Check sheet for the modelled part. Datum: model origin and axes. Units: mm. A direction names the side the tool comes from. Give positions to 0.01 mm unless a question says otherwise; leave off trailing zeros. Write each loop counter-clockwise with the first axis right and the second up, starting at its lowest first coordinate (ties: lowest second). Pieces come first, ordered by that corner, then holes. Notation, with made-up numbers: (53.5, 31) -> (74.5, 31) arc R17 ccw to (74.5, 35) -> close; hole circle Ø11 at (-9, -35). An arc over 180 degrees is marked (long way). Return JSON: item names as keys, results as strings.
from build123d import *

# Parameters (mm, degrees)
F1_DEPTH  = 26
F3_DEPTH  = 23
F4_W      = 86
F4_H      = 66
F5_DEPTH  = 5
F6_R      = 3
F7_R      = 3
F9_R      = 0.95
F10_DEPTH = 6


with BuildPart() as f1:
    # F0 (on Top) → F1 (new body)
    with BuildSketch(Plane.XY):
        with BuildLine():
            Line((76, 0), (10, 0))
            ThreePointArc((10, 0), (2.928932, -2.928932), (0, -10))
            Line((0, -10), (0, -56))
            ThreePointArc((0, -56), (2.928932, -63.071068), (10, -66))
            Line((10, -66), (76, -66))
            ThreePointArc((76, -66), (83.071068, -63.071068), (86, -56))
            Line((86, -56), (86, -10))
            ThreePointArc((86, -10), (83.071068, -2.928932), (76, 0))
        make_face()
    extrude(amount=F1_DEPTH)

    # F2 (on face) → F3 (cut)
    with BuildSketch(Plane.XY.offset(26)):
        with BuildLine():
            Line((73, -3), (13, -3))
            ThreePointArc((13, -3), (5.928932, -5.928932), (3, -13))
            Line((3, -13), (3, -53))
            ThreePointArc((3, -53), (5.928932, -60.071068), (13, -63))
            Line((13, -63), (73, -63))
            ThreePointArc((73, -63), (80.071068, -60.071068), (83, -53))
            Line((83, -53), (83, -13))
            ThreePointArc((83, -13), (80.071068, -5.928932), (73, -3))
        make_face()
    extrude(amount=-F3_DEPTH, mode=Mode.SUBTRACT)

    # F4 (on face) → F5 (cut)
    with BuildSketch(Plane.XY.offset(26)):
        with Locations((43, -33)):
            Rectangle(F4_W, F4_H)
        with BuildLine():
            ThreePointArc((1.5, -11.5), (4.428932, -4.428932), (11.5, -1.5))
            Line((11.5, -1.5), (74.5, -1.5))
            ThreePointArc((74.5, -1.5), (81.571068, -4.428932), (84.5, -11.5))
            Line((84.5, -11.5), (84.5, -54.5))
            ThreePointArc((84.5, -54.5), (81.571068, -61.571068), (74.5, -64.5))
            Line((74.5, -64.5), (11.5, -64.5))
            ThreePointArc((11.5, -64.5), (4.428932, -61.571068), (1.5, -54.5))
            Line((1.5, -54.5), (1.5, -11.5))
        make_face(mode=Mode.SUBTRACT)
    extrude(amount=-F5_DEPTH, mode=Mode.SUBTRACT)

    # F6
    f6_edges = [f1.edges().sort_by_distance(p)[0] for p in [
        (83.071068, -2.928932, 0),
        (43, 0, 0),
        (2.928932, -2.928932, 0),
        (0, -33, 0),
        (2.928932, -63.071068, 0),
        (43, -66, 0),
        (83.071068, -63.071068, 0),
        (86, -33, 0),
    ]]
    fillet(f6_edges, radius=F6_R)

    # F7
    f7_edges = [f1.edges().sort_by_distance(p)[0] for p in [
        (43, -3, 3),
        (5.928932, -5.928932, 3),
        (3, -33, 3),
        (5.928932, -60.071068, 3),
        (43, -63, 3),
        (80.071068, -60.071068, 3),
        (83, -33, 3),
        (80.071068, -5.928932, 3),
    ]]
    fillet(f7_edges, radius=F7_R)

    # F9 (on offset) → F10 (cut, symmetric)
    with BuildSketch(Plane.YZ.offset(43)):
        with Locations((-1.5, 23.6)):
            Circle(F9_R)
        with Locations((-64.5, 23.6)):
            Circle(F9_R)
    extrude(amount=F10_DEPTH, both=True, mode=Mode.SUBTRACT)


solid = f1.part
(1) Thickness scan on L1, parallel to Y at x = 27, z = 21.75; L2, parallel to X at y = -20.5, z = 24.5; L3, parallel to X at y = -14.5, z = 8. Record the ranges inside material, lowest first.
Reply:
{"L1": "-64.5 to -63, -3 to -1.5", "L2": "1.5 to 3, 83 to 84.5", "L3": "0 to 3, 83 to 86"}
(2) Release check for a two-part mould opening along X. For faces 6 (the cylindrical face through (80.15, -6.01, 16.14)), 7 (the cylindrical face through (43.46, -65.1, 0.86)), 8 (the cylindrical face through (4.35, -4.51, 23.54)) record: pulls with the +X half, pulls with the -X half, needs draft (parallel to the pull), parting line crosses it, or undercut.
Reply:
{"face 6": "undercut", "face 7": "needs draft", "face 8": "pulls with the -X half"}
(3) Cross-section at B-B on y = -43. Enter the section's corners in (x, z), then the cut area to 3 significant figures.
Reply:
{"outline": "(0, 3) arc R3 ccw to (3, 0) -> (83, 0) arc R3 ccw to (86, 3) -> (86, 21) -> (84.5, 21) -> (84.5, 26) -> (83, 26) -> (83, 6) arc R3 cw to (80, 3) -> (6, 3) arc R3 cw to (3, 6) -> (3, 26) -> (1.5, 26) -> (1.5, 21) -> (0, 21) -> close", "area": "381 mm^2"}
(4) Cross-section at A-A on z = 14.5. Enter the section's corners in (x, y).
Reply:
{"outline": "(0, -56) arc R10 ccw to (10, -66) -> (76, -66) arc R10 ccw to (86, -56) -> (86, -10) arc R10 ccw to (76, 0) -> (10, 0) arc R10 ccw to (0, -10) -> close; hole (3, -53) arc R10 ccw to (13, -63) -> (73, -63) arc R10 ccw to (83, -53) -> (83, -13) arc R10 ccw to (73, -3) -> (13, -3) arc R10 ccw to (3, -13) -> close"}
(5) Set-up check for faces 1 (the flat face through (43, -64.5, 25)), 2 (the cylindrical face through (81.49, -4.35, 23.54)), 3 (the cylindrical face through (43.42, -62.14, 3.9)), 4 (the cylindrical face through (43.08, -63.55, 23.58)), 5 (the cylindrical face through (4.51, -61.65, 23.54)): record each of +Z, -Z, +X, -X, +Y, -Y from which the full face is reachable in a straight line by a thin tool's end or side.
Reply:
{"face 1": "+Z, +X, -X, -Y", "face 2": "+Z, +X, +Y", "face 3": "+Z", "face 4": "-Y", "face 5": "+Z, -X, -Y"}
(6) Depth check by flat-ended pin: pin 1 Ø4 at (y, z) = (-58.5, 4.5) entering from -X; pin 2 Ø6 at (y, z) = (-56.5, 22.5) entering from +X; pin 3 Ø2.5 at (x, z) = (38.5, 24) entering from +Y; pin 4 Ø4 at (y, z) = (-30.5, 23.5) entering from -X. Enter the tip coordinate at first touch or a pass-through.
Reply:
{"pin 1": "x = 0.01", "pin 2": "x = 86", "pin 3": "y = -1.5", "pin 4": "x = 1.5"}
(7) Cross-section at C-C on x = 46. Enter the section's corners in (y, z).
Reply:
{"outline": "(-66, 3) arc R3 ccw to (-63, 0) -> (-3, 0) arc R3 ccw to (0, 3) -> (0, 21) -> (-1.5, 21) -> (-1.5, 22.65) arc R0.95 cw to (-1.5, 24.55) -> (-1.5, 26) -> (-3, 26) -> (-3, 6) arc R3 cw to (-6, 3) -> (-60, 3) arc R3 cw to (-63, 6) -> (-63, 26) -> (-64.5, 26) -> (-64.5, 24.55) arc R0.95 cw to (-64.5, 22.65) -> (-64.5, 21) -> (-66, 21) -> close"}
(8) Cross-section at D-D on x = 17. Enter the section's corners in (y, z), then the cut area to 3 significant figures.
Reply:
{"outline": "(-66, 3) arc R3 ccw to (-63, 0) -> (-3, 0) arc R3 ccw to (0, 3) -> (0, 21) -> (-1.5, 21) -> (-1.5, 26) -> (-3, 26) -> (-3, 6) arc R3 cw to (-6, 3) -> (-60, 3) arc R3 cw to (-63, 6) -> (-63, 26) -> (-64.5, 26) -> (-64.5, 21) -> (-66, 21) -> close", "area": "321 mm^2"}
